Can you work these out from the model? Positions are in its coordinate system, mm. A direction names the side the tool comes from. Round coordinates to 2 decimals unless told otherwise and drop trailing zeros. Write each loop counter-clockwise with the first axis right and the second up, starting at its lowest first coordinate (ties: lowest second). Pieces come first, ordered by that corner, then holes. Notation, with made-up numbers: (26.5, -18.75) -> (61.5, -18.75) arc R34 cw to (61.5, 17.25) -> close; hole circle Ø5 at (-24, 70). An arc over 180 degrees is marked (long way). Use CSV: the item, a comma, the result in double quotes.
```python
from build123d import *

# Parameters (mm, degrees)
SKETCH1_W                  = 19.304
SKETCH1_H                  = 19.304
SKETCH1_W_2                = 16.764
SKETCH1_H_2                = 16.764
BOSS_EXTRUDE1_DEPTH        = 508
FILLET1_R                  = 1.27
F_1_0_228_DIAMETER_HOLE2_D = 5.7912
F_1_0_228_DIAMETER_HOLE3_D = 5.7912


with BuildPart() as part:
    # Sketch1 → Boss-Extrude1 (new body)
    with BuildSketch(Plane(origin=(0, 0, 0), x_dir=(1, 0, 0), z_dir=(0, 1, 0))):
        Rectangle(SKETCH1_W, SKETCH1_H)
        Rectangle(SKETCH1_W_2, SKETCH1_H_2, mode=Mode.SUBTRACT)
    extrude(amount=BOSS_EXTRUDE1_DEPTH)

    # Fillet1
    fillet1_edges = [part.edges().sort_by_distance(p)[0] for p in [
        (-8.382, 254, 8.382),
        (8.382, 254, 8.382),
        (8.382, 254, -8.382),
        (-8.382, 254, -8.382),
        (9.652, 254, 9.652),
        (-9.652, 254, 9.652),
        (-9.652, 254, -9.652),
        (9.652, 254, -9.652),
    ]]
    fillet(fillet1_edges, radius=FILLET1_R)

    # #1 (0.228) Diameter Hole2 (through all)
    with Locations(Plane.ZY.offset(9.652)):
        with Locations((0, 463.55), (0, 44.45), (0, 254)):
            Hole(F_1_0_228_DIAMETER_HOLE2_D / 2)

    # #1 (0.228) Diameter Hole3 (through all)
    with Locations(Plane(origin=(0, 0, -9.652), x_dir=(-1, 0, 0), z_dir=(0, 0, -1))):
        with Locations((0, 420.6875), (0, 87.3125)):
            Hole(F_1_0_228_DIAMETER_HOLE3_D / 2)


solid = part.part
```
Q1. If we mould it in two halves opening along X, with no side actions, what happens to faces 3 (the face through (9.652, 250, 0)), 4 (the face through (-9.652, 250, 0)), 5 (the face through (0, 250, 8.382)), 6 (the face through (-9, 0, 0))? For each: released by +X, released by -X, zero draft, split by the parting line, or undercut.
Resolved:
face 3,"released by +X"
face 4,"released by -X"
face 5,"undercut"
face 6,"zero draft"
Q2. Will these pins go through, and if not, where does the flat tip stop? P1, Ø7.5, axis at y = 463.55, z = 0, coming from the +X side; P2, Ø4.5, axis at x = 0, y = 420.69, coming from the +Z side.
Resolved:
P1,"stops at x = 9.65"
P2,"passes through"
Q3. Suppose I cut it at A-A (y = 383). Write out the boundary of the cut face in (x, z).
Resolved:
outline,"(-9.65, -8.38) arc R1.27 ccw to (-8.38, -9.65) -> (8.38, -9.65) arc R1.27 ccw to (9.65, -8.38) -> (9.65, 8.38) arc R1.27 ccw to (8.38, 9.65) -> (-8.38, 9.65) arc R1.27 ccw to (-9.65, 8.38) -> close; hole (-8.38, -7.11) arc R1.27 ccw to (-7.11, -8.38) -> (7.11, -8.38) arc R1.27 ccw to (8.38, -7.11) -> (8.38, 7.11) arc R1.27 ccw to (7.11, 8.38) -> (-7.11, 8.38) arc R1.27 ccw to (-8.38, 7.11) -> close"
Q4. On a 3-axis mill with a long thin cutter (end or side, diameter ignored), from which of +Z, -Z, +X, -X, +Y, -Y can I reach the whole of each face in a straight line? I mean faces 1 (the face through (0, 250, 9.652)), 2 (the face through (8.382, 250, 0)). Say none if no direction works.
Resolved:
face 1,"+Z, +X, -X, +Y, -Y"
face 2,"+Y, -Y"
Q5. Please list where these lines run through material, in increasing order: probe 1 along Y at (x, z) = (0, 9.05); probe 2 along Y at (x, z) = (-9.35, 0); probe 3 along Z at (x, y) = (8.85, 254).
Resolved:
probe 1,"y = 0 to 84.42, 90.21 to 417.79, 423.58 to 508"
probe 2,"y = 0 to 41.55, 47.35 to 251.1, 256.9 to 460.65, 466.45 to 508"
probe 3,"z = -9.56 to -2.9, 2.9 to 9.56"
